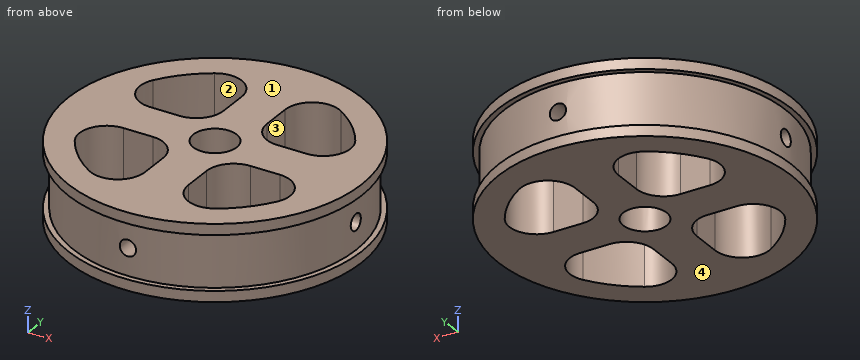
from build123d import *

# Parameters (mm, degrees)
ESQUISSE1_R             = 27
BOSS_EXTRU_1_DEPTH      = 2
ESQUISSE2_R             = 26
BOSS_EXTRU_2_DEPTH      = 10
ESQUISSE3_R             = 27
BOSS_EXTRU_3_DEPTH      = 2
ESQUISSE4_R             = 4
ENL_V_MAT_EXTRU_1_DEPTH = 41.669398815
ENL_V_MAT_EXTRU_2_DEPTH = 41.669398815
ESQUISSE6_R             = 1.5
ENL_V_MAT_EXTRU_3_DEPTH = 62.10646447
ESQUISSE7_R             = 1.5
ENL_V_MAT_EXTRU_4_DEPTH = 62.106464493


with BuildPart() as part:
    # Esquisse1 → Boss.-Extru.1 (new body)
    with BuildSketch(Plane.XY):
        Circle(ESQUISSE1_R)
    extrude(amount=BOSS_EXTRU_1_DEPTH)

    # Esquisse2 → Boss.-Extru.2 (add)
    with BuildSketch(Plane.XY.offset(2)):
        Circle(ESQUISSE2_R)
    extrude(amount=BOSS_EXTRU_2_DEPTH)

    # Esquisse3 → Boss.-Extru.3 (add)
    with BuildSketch(Plane.XY.offset(12)):
        Circle(ESQUISSE3_R)
    extrude(amount=BOSS_EXTRU_3_DEPTH)

    # Esquisse4 → Enlèv. mat.-Extru.1 (cut, through all)
    with BuildSketch(Plane.XY.offset(14)):
        Circle(ESQUISSE4_R)
    extrude(amount=-ENL_V_MAT_EXTRU_1_DEPTH, mode=Mode.SUBTRACT)

    # Esquisse5 → Enlèv. mat.-Extru.2 (cut, through all)
    with BuildSketch(Plane.XY.offset(14)):
        with BuildLine():
            Line((-4, 14.422205102), (-4, 9))
            ThreePointArc((-4, 9), (-5.464466094, 5.464466094), (-9, 4))
            Line((-9, 4), (-14.422205102, 4))
            ThreePointArc((-14.422205102, 4), (-18.794578263, 6.57464375), (-18.664030132, 11.647058824))
            ThreePointArc((-18.664030132, 11.647058824), (-15.556349186, 15.556349186), (-11.647058824, 18.664030132))
            ThreePointArc((-11.647058824, 18.664030132), (-6.57464375, 18.794578263), (-4, 14.422205102))
        make_face()
        with BuildLine():
            Line((4, 14.422205102), (4, 9))
            ThreePointArc((4, 9), (5.464466094, 5.464466094), (9, 4))
            Line((9, 4), (14.422205102, 4))
            ThreePointArc((14.422205102, 4), (18.794578263, 6.57464375), (18.664030132, 11.647058824))
            ThreePointArc((18.664030132, 11.647058824), (15.556349186, 15.556349186), (11.647058824, 18.664030132))
            ThreePointArc((11.647058824, 18.664030132), (6.57464375, 18.794578263), (4, 14.422205102))
        make_face()
        with BuildLine():
            Line((14.422205102, -4), (9, -4))
            ThreePointArc((9, -4), (5.464466094, -5.464466094), (4, -9))
            Line((4, -9), (4, -14.422205102))
            ThreePointArc((4, -14.422205102), (6.57464375, -18.794578263), (11.647058824, -18.664030132))
            ThreePointArc((11.647058824, -18.664030132), (15.556349186, -15.556349186), (18.664030132, -11.647058824))
            ThreePointArc((18.664030132, -11.647058824), (18.794578263, -6.57464375), (14.422205102, -4))
        make_face()
        with BuildLine():
            Line((-4, -9), (-4, -14.422205102))
            ThreePointArc((-4, -14.422205102), (-6.57464375, -18.794578263), (-11.647058824, -18.664030132))
            ThreePointArc((-11.647058824, -18.664030132), (-15.556349186, -15.556349186), (-18.664030132, -11.647058824))
            ThreePointArc((-18.664030132, -11.647058824), (-18.794578263, -6.57464375), (-14.422205102, -4))
            Line((-14.422205102, -4), (-9, -4))
            ThreePointArc((-9, -4), (-5.464466094, -5.464466094), (-4, -9))
        make_face()
    extrude(amount=-ENL_V_MAT_EXTRU_2_DEPTH, mode=Mode.SUBTRACT)

    # Esquisse6 → Enlèv. mat.-Extru.3 (cut, through all)
    with BuildSketch(Plane(origin=(0, 26, 0), x_dir=(-1, 0, 0), z_dir=(0, 1, 0))):
        with Locations((0, 7)):
            Circle(ESQUISSE6_R)
    extrude(amount=-ENL_V_MAT_EXTRU_3_DEPTH, mode=Mode.SUBTRACT)

    # Esquisse7 → Enlèv. mat.-Extru.4 (cut, through all)
    with BuildSketch(Plane.ZY.offset(26)):
        with Locations(Location((7, 0, 0), (0, 0, 270))):
            Circle(ESQUISSE7_R)
    extrude(amount=-ENL_V_MAT_EXTRU_4_DEPTH, mode=Mode.SUBTRACT)


solid = part.part
Can you work these out from the model? Positions are in its coordinate system, mm. Face numbers are marked on the shaded views. A direction names the side the tool comes from. Give positions to 0.01 mm unless a question says otherwise; leave off trailing zeros. Loops run counter-clockwise (first coordinate to the right, second up) from the corner with the lowest first, then second, coordinate; pieces in that order, holes last. Notation, with made-up numbers: M 19,32.25 L 54,32.25 A22 ccw 54,49.25 Z; hole C 31.25,61.5 d3. An arc over 180 degrees is marked long. One line per item, written item: value.
1) Imagine slicing it at A-A on y = 0. Write out the boundary of the cut face in (x, z).
Geometry check:
outline: M -27,0 L -4,0 L -4,5.5 L -26,5.5 L -26,2 L -27,2 Z; M -27,12 L -26,12 L -26,8.5 L -4,8.5 L -4,14 L -27,14 Z; M 4,0 L 27,0 L 27,2 L 26,2 L 26,5.5 L 4,5.5 Z; M 4,8.5 L 26,8.5 L 26,12 L 27,12 L 27,14 L 4,14 Z
2) Imagine slicing it at C-C on y = -5.5. Write out the boundary of the cut face in (x, z).
Geometry check:
outline: M -26.43,0 L -17.99,0 L -17.99,14 L -26.43,14 L -26.43,12 L -25.41,12 L -25.41,2 L -26.43,2 Z; M -5.43,0 L 5.43,0 L 5.43,14 L -5.43,14 Z; M 17.99,0 L 26.43,0 L 26.43,2 L 25.41,2 L 25.41,12 L 26.43,12 L 26.43,14 L 17.99,14 Z; hole C 0,7 d3
3) Imagine slicing it at B-B on x = 10. Write out the boundary of the cut face in (y, z), and give its area (3 significant figures).
Geometry check:
outline: M -25.08,0 L -19.32,0 L -19.32,14 L -25.08,14 L -25.08,12 L -24,12 L -24,2 L -25.08,2 Z; M -4,0 L 4,0 L 4,14 L -4,14 Z; M 19.32,0 L 25.08,0 L 25.08,2 L 24,2 L 24,12 L 25.08,12 L 25.08,14 L 19.32,14 Z; hole C 0,7 d3
area: 245 mm²
4) On a 3-axis mill with a long thin cutter (end or side, diameter ignored), from which of +Z, -Z, +X, -X, +Y, -Y can I reach the whole of each face in a straight line? I mean the marked faces 1 and 2. Say none if no direction works.
Geometry check:
face 1: +Z, +X, -X, +Y, -Y
face 2: +Z, -Z
5) Thinking about a two-plate mould opening in Y: for the marked faces 3 and 4, which applies, +Y half, -Y half, draft (parallel to the pull), parting line (faces both ways), or undercut?
Geometry check:
face 3: undercut
face 4: draft
6) Please list where these lines run through material, in increasing order: line 1 (Z direction, x = 20, y = 0); line 2 (X direction, y = -13.5, z = 7); line 3 (Y direction, x = -16.75, z = 7).
Geometry check:
line 1: z = 0 to 5.5, 8.5 to 14
line 2: x = -22.22 to -17.37, -4 to -1.5, 1.5 to 4, 17.37 to 22.22
line 3: y = -19.89 to -14.26, -4.57 to -1.5, 1.5 to 4.57, 14.26 to 19.89
7) I'm going to push flat-ended pins straight in: pin 1 (2 mm diameter, centred on x = 11, z = 3.5, fed in from +Y); pin 2 (2.5 mm diameter, centred on x = -11, z = 6.5, fed in from -Y); pin 3 (3.5 mm diameter, centred on y = 0, z = 7, fed in from -X); pin 4 (1 mm diameter, centred on x = 21, y = -20.5, fed in from +Z). Where does each tip first touch, or does it pass through?
Geometry check:
pin 1: stops at y = 24
pin 2: stops at y = -24.1
pin 3: stops at x = -26
pin 4: passes through
